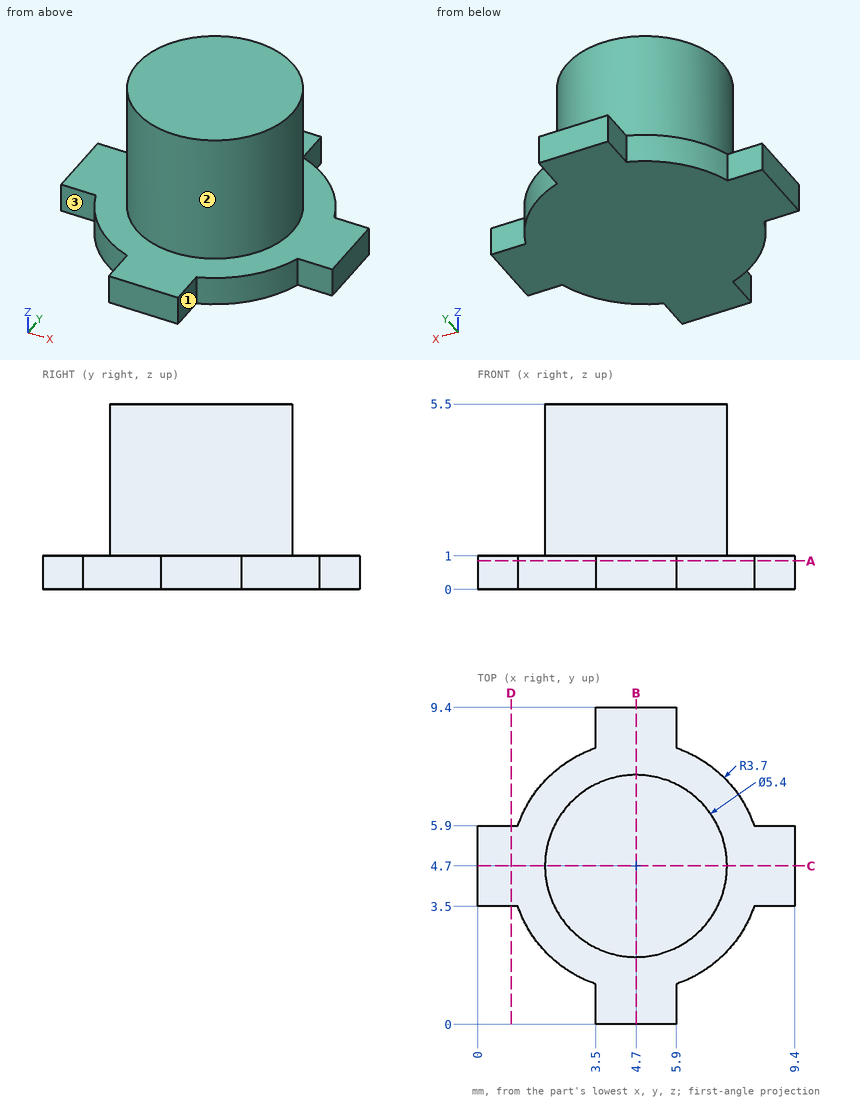
Study the drawing (mm; zero at the part's minimum x, y, z) and answer. A direction names the side the tool comes from. Give positions to 0.01 mm unless a question says otherwise; leave off trailing zeros. Loops run counter-clockwise (first coordinate to the right, second up) from the corner with the lowest first, then second, coordinate; pieces in that order, holes last. Notation, with made-up numbers: (36, 80) - (58, 80) arc R8 cw to (58, 93) - close; hole circle Ø5 at (-6.75, -16). An arc over 180 degrees is marked (long way). Return JSON: item names as keys, results as strings. Group by question number.
1. Find section A-A (z = 0.85). Write down the section's boundary in (x, y).
2. Which of the six approach directions +Z, -Z, +X, -X, +Y, -Y give full straight-line access (tool end or side, diameter ignored) to the marked faces 1, 2 and 3?
3. Straight lines are drawn through the part: line 1 (Z direction, x = 5.5, y = 9.25); line 2 (X direction, y = 8.5, z = 0.85); line 3 (X direction, y = 4, z = 5). For each, find the intervals that lie inside material, in ascending order. Write a range as [from, to].
4. Find section D-D (x = 1). Write down the section's boundary in (y, z), then the cut area to 3 significant figures.
5. Given pin 1 Ø1.1 at (y, z) = (0.5, 0.5) entering from -X; pin 2 Ø1.1 at (y, z) = (0.5, 0.5) entering from +X; pin 3 Ø1 at (x, z) = (2.5, 3) entering from -Y, each flat-ended and moving along its own axis, determine where each tip first touches the part or whether it passes through.
6. Find section B-B (x = 4.7). Write down the section's boundary in (y, z), then the cut area to 3 significant figures.
Verdict:
{
 "1": {"outline": "(0, 3.5) - (1.2, 3.5) arc R3.7 ccw to (3.5, 1.2) - (3.5, 0) - (5.9, 0) - (5.9, 1.2) arc R3.7 ccw to (8.2, 3.5) - (9.4, 3.5) - (9.4, 5.9) - (8.2, 5.9) arc R3.7 ccw to (5.9, 8.2) - (5.9, 9.4) - (3.5, 9.4) - (3.5, 8.2) arc R3.7 ccw to (1.2, 5.9) - (0, 5.9) - close"},
 "2": {"face 1": "+Z, -Z, +X, -Y", "face 2": "+Z", "face 3": "+Z, -Z, -X, -Y"},
 "3": {"line 1": "z = [0, 1]", "line 2": "x = [3.5, 5.9]", "line 3": "x = [2.09, 7.31]"},
 "4": {"outline": "(3.5, 0) - (5.9, 0) - (5.9, 1) - (3.5, 1) - close", "area": "2.40 mm^2"},
 "5": {"pin 1": "stops at x = 3.5", "pin 2": "stops at x = 5.9", "pin 3": "stops at y = 2.6"},
 "6": {"outline": "(0, 0) - (9.4, 0) - (9.4, 1) - (7.4, 1) - (7.4, 5.5) - (2, 5.5) - (2, 1) - (0, 1) - close", "area": "33.7 mm^2"}
}
